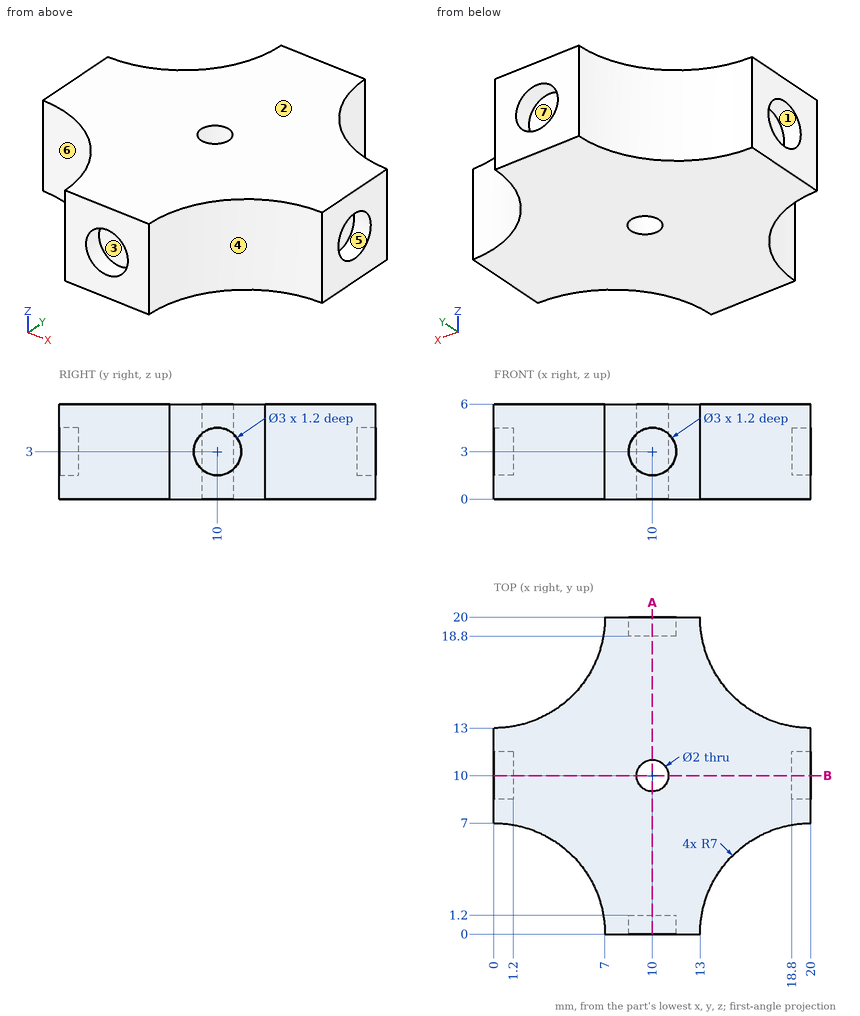
Source: three-view drawing plus pictorial views. Frame: mm from the lowest corner of the part. A direction names the side the tool comes from. Round coordinates to 2 decimals unless told otherwise and drop trailing zeros. Loops run counter-clockwise (first coordinate to the right, second up) from the corner with the lowest first, then second, coordinate; pieces in that order, holes last.
1. Ray query, L1, parallel to Y at x = 10, z = 3.35; L2, parallel to Z at x = 19.25, y = 10. Return the intervals inside material, ascending.
2. Mould query, pull axis X, two halves, no side actions, for the marked faces 4, 5, 6 and 7. Classes: released by +X, released by -X, zero draft, split by the parting line, or undercut.
3. Contact query for flat-ended pins moving along their axis: pin 1 (1.5 mm diameter, centred on x = 10.5, z = 2.5, fed in from +Y); pin 2 (3.5 mm diameter, centred on y = 10.5, z = 3, fed in from -X); pin 3 (1.6 mm diameter, centred on x = 10, y = 10, fed in from +Z); pin 4 (3 mm diameter, centred on x = 4.5, z = 5, fed in from -Y) (1 decimal). Output: stop coordinate, or through.
4. Section query A-A on x = 10. Output: boundary loops of the cut face in (y, z), and give its area (3 significant figures).
5. Access query for the marked faces 1, 2 and 3. Directions: +Z, -Z, +X, -X, +Y, -Y. A direction counts if a zero-diameter tool reaches every point of the face in a straight line with its end or side. Return the directions, or none.
Answers below:
1. L1: y = 1.2 to 9, 11 to 18.8
1. L2: z = 0 to 1.5, 4.5 to 6
2. face 4: released by +X
2. face 5: zero draft
2. face 6: released by -X
2. face 7: undercut
3. pin 1: stops at y = 18.8
3. pin 2: stops at x = 0
3. pin 3: passes through
3. pin 4: stops at y = 3.6
4. outline: (0, 0) - (9, 0) - (9, 6) - (0, 6) - (0, 4.5) - (1.2, 4.5) - (1.2, 1.5) - (0, 1.5) - close; (11, 0) - (20, 0) - (20, 1.5) - (18.8, 1.5) - (18.8, 4.5) - (20, 4.5) - (20, 6) - (11, 6) - close
4. area: 101 mm2
5. face 1: -X
5. face 2: +Z, +X, -X, +Y, -Y
5. face 3: -Y
